CAD build for the part. Positions are in the model's coordinates, mm. Face numbers are marked on the shaded views. A direction names the side the tool comes from. Coordinates: 2 decimals unless noted, no trailing zeros. Order: outer loops, then holes, each group sorted by start corner. A loop starts at its lowest first (then second) coordinate and runs counter-clockwise, first axis right, second up. Notation, with made-up numbers: M 14,-1.5 L 44,-1.5 A31 ccw 44,23.5 Z; hole C -8.75,-18.5 d5. An arc over 180 degrees is marked long. Write item = value, one per line.
from build123d import *

# Parameters (mm, degrees)
SKETCH_R      = 1.4
SKETCH_R_2    = 2
SKETCH_R_3    = 0.55
PAD_DEPTH     = 2
SKETCH001_R   = 2.5
SKETCH001_R_2 = 2
SKETCH001_R_3 = 2.25
SKETCH001_R_4 = 1.4
PAD001_DEPTH  = 2


with BuildPart() as part:
    # Sketch → Pad (new body)
    with BuildSketch(Plane.XY):
        Polygon((0, 10), (0, -10), (-8, -10), (-10.5, -12.5), (-28, -12.5), (-28, 12.5), (-10.5, 12.5), (-8, 10), align=None)
        with Locations((-6, 7)):
            Circle(SKETCH_R, mode=Mode.SUBTRACT)
        with Locations((-6, -7)):
            Circle(SKETCH_R, mode=Mode.SUBTRACT)
        with Locations((-25, -9.5)):
            Circle(SKETCH_R_2, mode=Mode.SUBTRACT)
        with Locations((-22, 0)):
            Circle(SKETCH_R_3, mode=Mode.SUBTRACT)
        with Locations((-19.46, 0)):
            Circle(SKETCH_R_3, mode=Mode.SUBTRACT)
        with BuildLine():
            ThreePointArc((-20.80911, 4.9), (-23, 10.9), (-25.19089, 4.9))
            Line((-25.19089, 4.9), (-20.80911, 4.9))
        make_face(mode=Mode.SUBTRACT)
    extrude(amount=PAD_DEPTH)

    # Sketch001 (on DatumPlane) → Pad001 (join)
    with BuildSketch(Plane.XY.offset(2)):
        with Locations((-25, -9.5)):
            Circle(SKETCH001_R)
        with Locations((-25, -9.5)):
            Circle(SKETCH001_R_2, mode=Mode.SUBTRACT)
        with Locations((-6, -7)):
            Circle(SKETCH001_R_3)
        with Locations((-6, -7)):
            Circle(SKETCH001_R_4, mode=Mode.SUBTRACT)
        with Locations((-6, 7)):
            Circle(SKETCH001_R_3)
        with Locations((-6, 7)):
            Circle(SKETCH001_R_4, mode=Mode.SUBTRACT)
    extrude(amount=PAD001_DEPTH)


solid = part.part
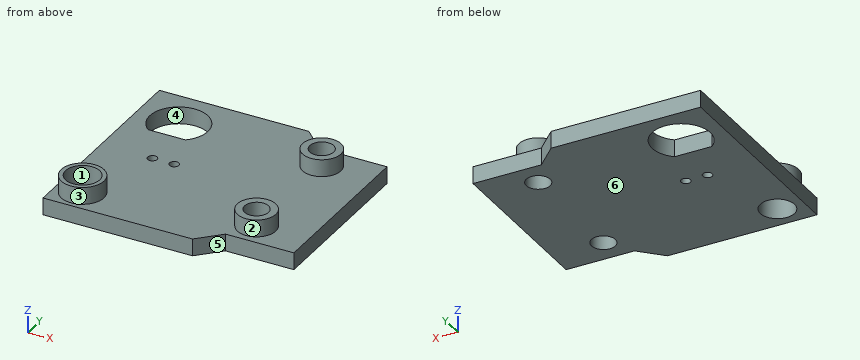
(1) Tool access for the marked faces 1 and 2: list every direction of +Z, -Z, +X, -X, +Y, -Y with a clear straight run to the whole face (end or side of a thin tool).
Evaluation:
face_1 = +Z, -Z
face_2 = +Z
(2) Slice it at B-B, the plane z = 2.45. Write the cut outline in (x, y), then the cut area to 3 significant figures.
Evaluation:
outline = C -25,-9.5 d5; C -6,-7 d4.5; C -6,7 d4.5; hole C -25,-9.5 d4; hole C -6,-7 d2.8; hole C -6,7 d2.8
area = 26.6 mm²
(3) Slice it at C-C, the plane y = 0. Write the cut outline in (x, z).
Evaluation:
outline = M -28,0 L -22.55,0 L -22.55,2 L -28,2 Z; M -21.45,0 L -20.01,0 L -20.01,2 L -21.45,2 Z; M -18.91,0 L 0,0 L 0,2 L -18.91,2 Z
(4) Slice it at D-D, the plane z = 0.6. Write the cut outline in (x, y).
Evaluation:
outline = M -28,-12.5 L -10.5,-12.5 L -8,-10 L 0,-10 L 0,10 L -8,10 L -10.5,12.5 L -28,12.5 Z; hole C -25,-9.5 d4; hole M -25.19,4.9 L -20.81,4.9 A3.4 ccw long Z; hole C -22,0 d1.1; hole C -19.46,0 d1.1; hole C -6,-7 d2.8; hole C -6,7 d2.8
(5) Pull direction X, two halves, no side cores. Call the marked faces 3, 4, 5 and 6: +X half, -X half, draft (parallel to the pull), parting line (faces both ways), or undercut.
Evaluation:
face_3 = undercut
face_4 = undercut
face_5 = +X half
face_6 = draft
(6) Wall check: line 1 (Y direction, x = -6, z = 1.4); line 2 (Y direction, x = -6, z = 3.05); line 3 (Y direction, x = -19.46, z = 1.05). Give the ranges that are in metal, low to high. Write a range as from..to.
Evaluation:
line_1 = -10..-8.4, -5.6..5.6, 8.4..10
line_2 = -9.25..-8.4, -5.6..-4.75, 4.75..5.6, 8.4..9.25
line_3 = -12.5..-0.55, 0.55..12.5
(7) Slice it at A-A, the plane x = -6. Write the cut outline in (y, z).
Evaluation:
outline = M -10,0 L -8.4,0 L -8.4,4 L -9.25,4 L -9.25,2 L -10,2 Z; M -5.6,0 L 5.6,0 L 5.6,4 L 4.75,4 L 4.75,2 L -4.75,2 L -4.75,4 L -5.6,4 Z; M 8.4,0 L 10,0 L 10,2 L 9.25,2 L 9.25,4 L 8.4,4 Z
(8) Pin check, flat tips, straight feed: pin 1 Ø1.4 at (x, y) = (-22, 0) entering from +Z; pin 2 Ø2 at (x, z) = (-7, 3.5) entering from +Y; pin 3 Ø0.6 at (x, z) = (-2.5, 1.5) entering from +Y. Stop position of each tip, or through.
Evaluation:
pin_1 = 2
pin_2 = 9.25
pin_3 = 10
